from build123d import *

# Parameters (mm, degrees)
F2_R     = 3.5634649621
F3_DEPTH = 25.4
F4_DEPTH = 25.4


with BuildPart() as f1:
    # F0 (on Front) → F1 (revolve)
    with BuildSketch(Plane.XZ):
        with BuildLine():
            Line((0, -31.6168554127), (0, 14.6877852364))
            Line((0, 14.6877852364), (0, 41.4482640938))
            add(Edge.make_bspline(
                [(0, 41.4482640938), (-25.6740520635, 41.4482640938), (-16.1890444672, 23.12483641)],
                knots=[1.5707963268, 1.5707963268, 1.5707963268, 3.5199983734, 3.5199983734, 3.5199983734], degree=2, weights=[1, 0.5614982427, 1]))
            ThreePointArc((-16.1890444672, 23.12483641), (-26.1269124398, 12.7069231562), (-19.3572565913, 0))
            ThreePointArc((-19.3572565913, 0), (-31.9139919734, 0.5656111198), (-43.2330009959, 6.0310986683))
            ThreePointArc((-43.2330009959, 6.0310986683), (-53.884249017, 4.6653287196), (-63.5563284159, 0))
            ThreePointArc((-63.5563284159, 0), (-61.1052161076, -1.5398735842), (-58.5253632579, -2.852703153))
            ThreePointArc((-58.5253632579, -2.852703153), (-47.4894028022, 0.7494839504), (-37.2366299676, -4.6955894476))
            ThreePointArc((-37.2366299676, -4.6955894476), (-34.7183947898, -3.9333720133), (-32.2710320848, -2.9675047252))
            ThreePointArc((-32.2710320848, -2.9675047252), (-26.3415646355, -9.3488473307), (-18.0822180019, -12.1171158992))
            add(Edge.make_bspline(
                [(-18.0822180019, -12.1171158992), (-18.0762251984, -12.3795353184), (-17.9455253082, -18.958346138), (-18.6461523511, -28.5006584635), (-12.0803813525, -30.8886451777), (-9.6367610934, -31.2720729229)],
                knots=[0.4937011161, 0.4937011161, 0.4937011161, 0.4937011161, 0.5040536134, 0.7530494568, 0.866814487, 0.866814487, 0.866814487, 0.866814487], degree=3))
            Line((-9.6367610934, -31.2720729229), (-9.0325408773, -31.2720729229))
            Line((-9.0325408773, -31.2720729229), (-9.0325408773, -31.3586124199))
            add(Edge.make_bspline(
                [(-9.0325408773, -31.3586124199), (-6.3048687908, -31.7137212723), (-3.1526142589, -31.6653227611), (0, -31.6168554127)],
                knots=[0.8760752846, 0.8760752846, 0.8760752846, 0.8760752846, 1, 1, 1, 1], degree=3))
        make_face()
        with BuildLine():
            Line((0, -37.4240316451), (0, -31.6168554127))
            add(Edge.make_bspline(
                [(-9.0325408773, -31.3586124199), (-6.3048687908, -31.7137212723), (-3.1526142589, -31.6653227611), (0, -31.6168554127)],
                knots=[0.8760752846, 0.8760752846, 0.8760752846, 0.8760752846, 1, 1, 1, 1], degree=3))
            Line((-9.0325408773, -31.3586124199), (-9.0325408773, -53.8723139956))
            Line((-9.0325408773, -53.8723139956), (-4.5162704386, -53.8723139956))
            Line((-4.5162704386, -53.8723139956), (0, -37.4240316451))
        make_face()
    revolve(axis=Axis((0, 0, 2.0121162244), (0, 0, -1)))

    # F2 (on Right) → F3 (cut)
    with BuildSketch(Plane.YZ):
        with Locations((0, -43.2312116027)):
            Circle(F2_R)
    extrude(amount=-F3_DEPTH, mode=Mode.SUBTRACT)

    # F2 (on Right) → F4 (cut)
    with BuildSketch(Plane.YZ):
        with Locations((0, -43.2312116027)):
            Circle(F2_R)
    extrude(amount=F4_DEPTH, mode=Mode.SUBTRACT)


solid = f1.part
Input: part model. Units: mm. Frame: model coordinates. Round coordinates to 2 decimals unless told otherwise and drop trailing zeros. Order: outer loops, then holes, each group sorted by start corner. A loop starts at its lowest first (then second) coordinate and runs counter-clockwise, first axis right, second up. Notation, with made-up numbers: (18.25, 85) - (68.25, 85) arc R20 cw to (68.25, 100) - close; hole circle Ø4 at (-30.5, 79). An arc over 180 degrees is marked (long way). Answer as a JSON object with one key per item and string values. Group by question number.
(1) Pin query (flat end, axial travel): P1, Ø5, axis at x = -40.5, y = -8.5, coming from the +Z side; P2, Ø5, axis at y = 47.5, z = 9.5, coming from the -X side; P3, Ø10, axis at y = -13.5, z = 18.5, coming from the -X side; P4, Ø9.5, axis at y = 0, z = -43.23, coming from the -X side. Return the tip coordinate at first contact, or that it passes through.
(2) Cut plane A-A (z = 10). Return loops of the section in (x, y), then the cut area to 3 significant figures.
(3) Draft query along Y for faces 1 (the face through (0.13, 1.92, -40.23)), 2 (the face through (-4.168, -8.013, -42.73)), 3 (the face through (-4, -4, -53.872)). Return one class per face: released by +Y, released by -Y, zero draft, split by the parting line, or undercut.
(4) Material intervals for probe 1 along Z at (x, y) = (0, 16.5); probe 2 along Z at (x, y) = (1, 0); probe 3 along Z at (x, y) = (-30, -27.5) (3 decimals), sorted ascending. Write a range as from..to.
Here are the results:
{
 "1": {"P1": "stops at z = 6.05", "P2": "passes through", "P3": "stops at x = -23.58", "P4": "stops at x = -9.03"},
 "2": {"outline": "circle Ø52.39 at (0, 0)", "area": "2,160 mm^2"},
 "3": {"face 1": "undercut", "face 2": "split by the parting line", "face 3": "zero draft"},
 "4": {"probe 1": "z = -27.28..23.06, 23.77..32.36", "probe 2": "z = -39.67..41.43", "probe 3": "z = -1.583..4.285"}
}
